```python
from build123d import *

# Parameters (mm, degrees)
F1_DEPTH = 1.5


with BuildPart() as f1:
    # F0 (on Top) → F1 (new body, symmetric)
    with BuildSketch(Plane.XY):
        Polygon((-52.603185, 89.276404), (-52.603174, 86.276474), (-55.603174, 86.276415), (-55.603174, 6.276474), (-52.603185, 6.276474), (-52.603185, 3.276485), (-34.603174, 3.276474), (-34.603174, 6.276474), (-31.603174, 6.276474), (-31.603174, 26.276474), (-42.603279, 26.276459), (-42.603279, 66.27643), (-31.603261, 66.27643), (-31.603261, 86.276415), (-34.603174, 86.276474), (-34.60325, 89.276404), align=None)
        with BuildLine():
            ThreePointArc((-47.353174, 30.276474), (-48.060281, 30.569367), (-48.353174, 31.276474))
            ThreePointArc((-48.353174, 31.276474), (-48.060281, 31.983581), (-47.353174, 32.276474))
            Line((-47.353174, 32.276474), (-45.853174, 32.276474))
            ThreePointArc((-45.853174, 32.276474), (-45.146067, 31.983581), (-44.853174, 31.276474))
            ThreePointArc((-44.853174, 31.276474), (-45.146067, 30.569367), (-45.853174, 30.276474))
            Line((-45.853174, 30.276474), (-47.353174, 30.276474))
        make_face(mode=Mode.SUBTRACT)
        with BuildLine():
            ThreePointArc((-47.353174, 40.276474), (-48.060281, 40.569367), (-48.353174, 41.276474))
            ThreePointArc((-48.353174, 41.276474), (-48.060281, 41.983581), (-47.353174, 42.276474))
            Line((-47.353174, 42.276474), (-45.853174, 42.276474))
            ThreePointArc((-45.853174, 42.276474), (-45.146067, 41.983581), (-44.853174, 41.276474))
            ThreePointArc((-44.853174, 41.276474), (-45.146067, 40.569367), (-45.853174, 40.276474))
            Line((-45.853174, 40.276474), (-47.353174, 40.276474))
        make_face(mode=Mode.SUBTRACT)
        with BuildLine():
            ThreePointArc((-36.353174, 10.276474), (-37.060281, 10.569367), (-37.353174, 11.276474))
            ThreePointArc((-37.353174, 11.276474), (-37.060281, 11.983581), (-36.353174, 12.276474))
            Line((-36.353174, 12.276474), (-34.853174, 12.276474))
            ThreePointArc((-34.853174, 12.276474), (-34.146067, 11.983581), (-33.853174, 11.276474))
            ThreePointArc((-33.853174, 11.276474), (-34.146067, 10.569367), (-34.853174, 10.276474))
            Line((-34.853174, 10.276474), (-36.353174, 10.276474))
        make_face(mode=Mode.SUBTRACT)
        with BuildLine():
            ThreePointArc((-36.353174, 20.276474), (-37.060281, 20.569367), (-37.353174, 21.276474))
            ThreePointArc((-37.353174, 21.276474), (-37.060281, 21.983581), (-36.353174, 22.276474))
            Line((-36.353174, 22.276474), (-34.853174, 22.276474))
            ThreePointArc((-34.853174, 22.276474), (-34.146067, 21.983581), (-33.853174, 21.276474))
            ThreePointArc((-33.853174, 21.276474), (-34.146067, 20.569367), (-34.853174, 20.276474))
            Line((-34.853174, 20.276474), (-36.353174, 20.276474))
        make_face(mode=Mode.SUBTRACT)
        with BuildLine():
            ThreePointArc((-47.353174, 50.276474), (-48.060281, 50.569367), (-48.353174, 51.276474))
            ThreePointArc((-48.353174, 51.276474), (-48.060281, 51.983581), (-47.353174, 52.276474))
            Line((-47.353174, 52.276474), (-45.853174, 52.276474))
            ThreePointArc((-45.853174, 52.276474), (-45.146067, 51.983581), (-44.853174, 51.276474))
            ThreePointArc((-44.853174, 51.276474), (-45.146067, 50.569367), (-45.853174, 50.276474))
            Line((-45.853174, 50.276474), (-47.353174, 50.276474))
        make_face(mode=Mode.SUBTRACT)
        with BuildLine():
            ThreePointArc((-47.353174, 60.276474), (-48.060281, 60.569367), (-48.353174, 61.276474))
            ThreePointArc((-48.353174, 61.276474), (-48.060281, 61.983581), (-47.353174, 62.276474))
            Line((-47.353174, 62.276474), (-45.853174, 62.276474))
            ThreePointArc((-45.853174, 62.276474), (-45.146067, 61.983581), (-44.853174, 61.276474))
            ThreePointArc((-44.853174, 61.276474), (-45.146067, 60.569367), (-45.853174, 60.276474))
            Line((-45.853174, 60.276474), (-47.353174, 60.276474))
        make_face(mode=Mode.SUBTRACT)
        with BuildLine():
            ThreePointArc((-36.353174, 70.276474), (-37.060281, 70.569367), (-37.353174, 71.276474))
            ThreePointArc((-37.353174, 71.276474), (-37.060281, 71.983581), (-36.353174, 72.276474))
            Line((-36.353174, 72.276474), (-34.853174, 72.276474))
            ThreePointArc((-34.853174, 72.276474), (-34.146067, 71.983581), (-33.853174, 71.276474))
            ThreePointArc((-33.853174, 71.276474), (-34.146067, 70.569367), (-34.853174, 70.276474))
            Line((-34.853174, 70.276474), (-36.353174, 70.276474))
        make_face(mode=Mode.SUBTRACT)
        with BuildLine():
            ThreePointArc((-36.353174, 80.276474), (-37.060281, 80.569367), (-37.353174, 81.276474))
            ThreePointArc((-37.353174, 81.276474), (-37.060281, 81.983581), (-36.353174, 82.276474))
            Line((-36.353174, 82.276474), (-34.853174, 82.276474))
            ThreePointArc((-34.853174, 82.276474), (-34.146067, 81.983581), (-33.853174, 81.276474))
            ThreePointArc((-33.853174, 81.276474), (-34.146067, 80.569367), (-34.853174, 80.276474))
            Line((-34.853174, 80.276474), (-36.353174, 80.276474))
        make_face(mode=Mode.SUBTRACT)
    extrude(amount=F1_DEPTH, both=True)


solid = f1.part
```
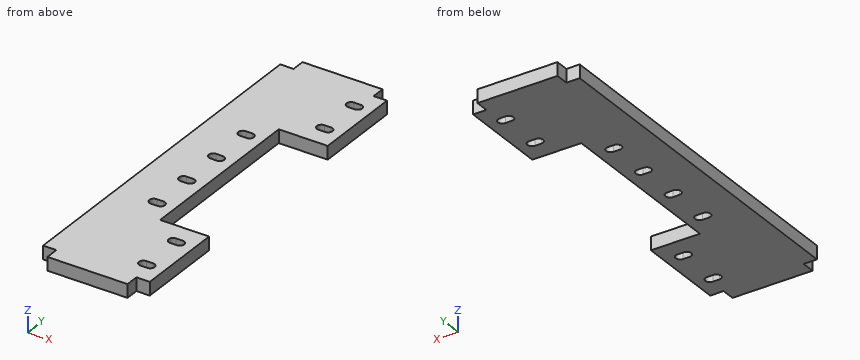
CAD build for the part. Positions are in the model's coordinates, mm. Round coordinates to 2 decimals unless told otherwise and drop trailing zeros. Loops run counter-clockwise (first coordinate to the right, second up) from the corner with the lowest first, then second, coordinate; pieces in that order, holes last. Notation, with made-up numbers: (-5, 2.25) - (21, 2.25) arc R29 cw to (21, 39.25) - close; hole circle Ø2 at (-26, 19.5). An arc over 180 degrees is marked (long way). Return JSON: item names as keys, results as strings. Group by question number.
Q1. Band-saw the part on A-A on z = -1. Give the number of separate pieces and of enclosed holes in the cut face, plus the area to 3 significant figures.
Q2. Drill centre lines: line 1 along Y through (x, z) = (-36.25, -0.2); line 2 along Y through (x, z) = (-39, 0.9); line 3 along X through (y, z) = (44.5, 1.4). Where is each one in solid material? Low to high. Write a range as [from, to].
Q3. Band-saw the part on B-B on y = 44.5. Give the cut face in (x, z), plus the area to 3 significant figures.
Q4. Flat gauge pin, fed straight in: pin 1 Ø0.9 at (y, z) = (38.5, 0.5) entering from +X. Where does the tip first touch, or does it go through?
Solutions:
{
 "1": {"separate pieces": "1", "enclosed holes": "8", "area": "1,540 mm^2"},
 "2": {"line 1": "y = [3.28, 10.28], [12.28, 20.28], [22.28, 26.28], [66.28, 70.28], [72.28, 80.28], [82.28, 89.28]", "line 2": "y = [3.28, 26.28], [66.28, 89.28]", "line 3": "x = [-55.6, -42.6]"},
 "3": {"outline": "(-55.6, -1.5) - (-42.6, -1.5) - (-42.6, 1.5) - (-55.6, 1.5) - close", "area": "39.0 mm^2"},
 "4": {"pin 1": "stops at x = -42.6"}
}
